```python
from build123d import *

# Parameters (mm, degrees)
F0_R          = 4.2
F0_R_2        = 23.5
F1_DEPTH      = 12
F3_R          = 40
F4_DEPTH      = 2
F4_DEPTH_BACK = 10
F6_D          = 5
F7_D          = 12


with BuildPart() as f1:
    # F0 (on Top) → F1 (new body)
    with BuildSketch(Plane.XY):
        with BuildLine():
            Line((75, 129.9038105677), (-75, 129.9038105677))
            ThreePointArc((-75, 129.9038105677), (-150, 0), (-75, -129.9038105677))
            Line((-75, -129.9038105677), (75, -129.9038105677))
            ThreePointArc((75, -129.9038105677), (150, 0), (75, 129.9038105677))
        make_face()
        with Locations((0, -110)):
            Circle(F0_R, mode=Mode.SUBTRACT)
        with Locations((-95.2627944163, -55)):
            Circle(F0_R, mode=Mode.SUBTRACT)
        with Locations((95.2627944163, -55)):
            Circle(F0_R, mode=Mode.SUBTRACT)
        with Locations((-95.2627944163, 55)):
            Circle(F0_R, mode=Mode.SUBTRACT)
        Circle(F0_R_2, mode=Mode.SUBTRACT)
        with Locations((0, 110)):
            Circle(F0_R, mode=Mode.SUBTRACT)
        with Locations((95.2627944163, 55)):
            Circle(F0_R, mode=Mode.SUBTRACT)
    extrude(amount=-F1_DEPTH)

    # F3 (on offset) → F4 (cut, two sides)
    with BuildSketch(Plane(origin=(0, 0, -12), x_dir=(1, 0, 0), z_dir=(0, 0, -1))) as f4_sk:
        Circle(F3_R)
    extrude(amount=-F4_DEPTH, mode=Mode.SUBTRACT)
    extrude(f4_sk.sketch, amount=F4_DEPTH_BACK, mode=Mode.SUBTRACT)

    # F6 (through all)
    with Locations(Plane(origin=(0, 0, -12), x_dir=(1, 0, 0), z_dir=(0, 0, -1))):
        with Locations((6.105887852, 31.4120698703), (-24.1507065671, 20.9938889277), (-30.2565944192, -10.4181809426), (-6.105887852, -31.4120698703), (24.1507065671, -20.9938889277), (30.2565944192, 10.4181809426)):
            Hole(F6_D / 2)

    # F7 (through all)
    with Locations(Plane(origin=(0, 0, -12), x_dir=(1, 0, 0), z_dir=(0, 0, -1))):
        with Locations((-30.8347743626, -35.4713502705), (15.3017032595, -44.4393730532), (46.136477622, -8.9680227827), (30.8347743626, 35.4713502705), (-15.3017032595, 44.4393730532), (-46.136477622, 8.9680227827)):
            Hole(F7_D / 2)


solid = f1.part
```
Input: part model. Units: mm. Frame: model coordinates. A direction names the side the tool comes from. Give positions to 0.01 mm unless a question says otherwise; leave off trailing zeros. Loops run counter-clockwise (first coordinate to the right, second up) from the corner with the lowest first, then second, coordinate; pieces in that order, holes last.
1) Line query: L1, parallel to X at y = 12, z = -2.25; L2, parallel to Y at x = 1, z = -3.25; L3, parallel to X at y = 13.5, z = -6.5. Output: solid intervals per line, ascending.
A:
L1: x = -149.52 to -32.19, -28.32 to -20.21, 20.21 to 40.96, 51.31 to 149.52
L2: y = -129.9 to -114.08, -105.92 to -23.48, 23.48 to 105.92, 114.08 to 129.9
L3: x = -149.39 to -19.24, 19.24 to 42.2, 50.07 to 149.39
2) Contact query for flat-ended pins moving along their axis: pin 1 (5 mm diameter, centred on y = -57.5, z = -9, fed in from +X); pin 2 (6 mm diameter, centred on x = -30.26, y = 10.42, fed in from -Z); pin 3 (2 mm diameter, centred on x = -100.5, z = -2.5, fed in from +Y). Output: stop coordinate, or through.
A:
pin 1: stops at x = 139.55
pin 2: stops at z = -10
pin 3: stops at y = 112.25
3) Mould query, pull axis X, two halves, no side actions, for faces 1 (the cylindrical face through (42.91, 3.91, -5.92)), 2 (the flat face through (-2, 31, 0)), 3 (the cylindrical face through (149.984, -2.199, -5.916)), 4 (the cylindrical face through (-26.41, 31.42, -5.92)). Classes: released by +X, released by -X, zero draft, split by the parting line, or undercut.
A:
face 1: undercut
face 2: zero draft
face 3: released by +X
face 4: undercut
4) Section query C-C on z = -3. Count the separate pieces of the cut face and the enclosed holes in it, and give its area (3 significant figures).
A:
separate pieces: 1
enclosed holes: 19
area: 63,700 mm2
5) Section query D-D on y = 55. Return the cut outline in (x, z), and give its area (3 significant figures).
A:
outline: (-139.55, -12) - (-99.46, -12) - (-99.46, 0) - (-139.55, 0) - close; (-91.06, -12) - (91.06, -12) - (91.06, 0) - (-91.06, 0) - close; (99.46, -12) - (139.55, -12) - (139.55, 0) - (99.46, 0) - close
area: 3,150 mm2
6) Reachability of faces 5 (the flat face through (17, 17, -10)), 6 (the cylindrical face through (-149.984, 2.199, -5.916)) from +Z, -Z, +X, -X, +Y, -Y: full face, straight path, thin tool, end or side. Return the list, or none.
A:
face 5: -Z
face 6: +Z, -Z, -X
7) Section query A-A on x = 0. Return the cut outline in (y, z).
A:
outline: (-129.9, -12) - (-114.2, -12) - (-114.2, 0) - (-129.9, 0) - close; (-105.8, -12) - (-40, -12) - (-40, -10) - (-23.5, -10) - (-23.5, 0) - (-105.8, 0) - close; (23.5, -10) - (40, -10) - (40, -12) - (105.8, -12) - (105.8, 0) - (23.5, 0) - close; (114.2, -12) - (129.9, -12) - (129.9, 0) - (114.2, 0) - close
8) Section query B-B on y = 110. Return the cut outline in (x, z).
A:
outline: (-101.98, -12) - (-4.2, -12) - (-4.2, 0) - (-101.98, 0) - close; (4.2, -12) - (101.98, -12) - (101.98, 0) - (4.2, 0) - close
